Check sheet for the modelled part. Datum: model origin and axes. Units: mm. Give positions to 0.01 mm unless a question says otherwise; leave off trailing zeros. Order: outer loops, then holes, each group sorted by start corner. A loop starts at its lowest first (then second) coordinate and runs counter-clockwise, first axis right, second up.
Item 1: Sectioned sample at B-B on z = 0.9. Count the separate pieces of the cut face and the enclosed holes in it, and give its area (3 significant figures).
Item 2: Sectioned sample at C-C on x = 22. Record the boundary of the cut face in (y, z), and give its area (3 significant figures).
Item 3: Release check for a two-part mould opening along Y. For faces 1 (the cylindrical face through (44.77, 25.99, 0.78)), 2 (the cylindrical face through (28.331, 44.323, 0.783)), 3 (the flat face through (0, 23, 1)) record: released by +Y, released by -Y, zero draft, split by the parting line, or undercut.
Item 4: Gauge pin test, flat end, axial feed: P1, Ø4, axis at x = 5.97, y = 42.72, coming from the +Z side. Record the tip position at first contact, or that the pin passes through.
Item 5: Material ranges on line 1 along X through (y, z) = (8, 1.5); line 2 along Y through (x, z) = (4.5, 0.3); line 3 along X through (y, z) = (27, 1.45), recorded low to high.
Item 6: Sectioned sample at A-A on y = 39.37. Record the boundary of the cut face in (x, z).
Item 7: Sectioned sample at D-D on x = 50. Record the boundary of the cut face in (y, z).
from build123d import *

# Parameters (mm, degrees)
F0_R     = 2.2987
F0_R_2   = 2.3876
F0_R_3   = 11.1125
F1_DEPTH = 1.5875


with BuildPart() as f1:
    # F0 (on Top) → F1 (new body)
    with BuildSketch(Plane.XY):
        with BuildLine():
            Line((0, 46.101), (0, 0))
            Line((0, 0), (56.388, 0))
            Line((56.388, 0), (56.388, 46.101))
            Line((56.388, 46.101), (38.6588, 46.101))
            ThreePointArc((38.6588, 46.101), (28.1813, 44.322395), (17.7038, 46.101))
            Line((17.7038, 46.101), (0, 46.101))
        make_face()
        with Locations((5.969, 7.7978)):
            Circle(F0_R, mode=Mode.SUBTRACT)
        with Locations((28.194, 10.9728)):
            Circle(F0_R_2, mode=Mode.SUBTRACT)
        with Locations((50.419, 7.7978)):
            Circle(F0_R, mode=Mode.SUBTRACT)
        with Locations((5.969, 42.7228)):
            Circle(F0_R, mode=Mode.SUBTRACT)
        with Locations((13.9192, 25.273)):
            Circle(F0_R_2, mode=Mode.SUBTRACT)
        with Locations((28.194, 25.273)):
            Circle(F0_R_3, mode=Mode.SUBTRACT)
        with Locations((42.4942, 25.273)):
            Circle(F0_R_2, mode=Mode.SUBTRACT)
        with Locations((28.194, 39.37)):
            Circle(F0_R_2, mode=Mode.SUBTRACT)
        with Locations((50.419, 42.7228)):
            Circle(F0_R, mode=Mode.SUBTRACT)
    extrude(amount=F1_DEPTH)


solid = f1.part
Report:
1. separate pieces: 1
1. enclosed holes: 9
1. area: 2,050 mm2
2. outline: (0, 0) - (16.05, 0) - (16.05, 1.59) - (0, 1.59) - close; (34.5, 0) - (44.93, 0) - (44.93, 1.59) - (34.5, 1.59) - close
2. area: 42.0 mm2
3. face 1: undercut
3. face 2: released by +Y
3. face 3: zero draft
4. P1: passes through
5. line 1: x = 0 to 3.68, 8.26 to 48.13, 52.71 to 56.39
5. line 2: y = 0 to 6.03, 9.57 to 40.95, 44.49 to 46.1
5. line 3: x = 0 to 12.27, 15.57 to 17.22, 39.17 to 40.85, 44.14 to 56.39
6. outline: (0, 0) - (25.81, 0) - (25.81, 1.59) - (0, 1.59) - close; (30.58, 0) - (56.39, 0) - (56.39, 1.59) - (30.58, 1.59) - close
7. outline: (0, 0) - (5.54, 0) - (5.54, 1.59) - (0, 1.59) - close; (10.06, 0) - (40.46, 0) - (40.46, 1.59) - (10.06, 1.59) - close; (44.98, 0) - (46.1, 0) - (46.1, 1.59) - (44.98, 1.59) - close
